Design review of the part shown in the three views and the two pictorial views. Dimensions are in mm from the part's minimum x, y and z. A direction names the side the tool comes from. Coordinates: 2 decimals unless noted, no trailing zeros. Order: outer loops, then holes, each group sorted by start corner. A loop starts at its lowest first (then second) coordinate and runs counter-clockwise, first axis right, second up. Notation, with made-up numbers: (-3.75, 59.5) -> (20.25, 59.5) arc R22 cw to (20.25, 67.5) -> close; hole circle Ø6 at (2.25, 22.5). An arc over 180 degrees is marked (long way). Answer as a JSON object with one key per item and string values. Group by question number.
1) Wall thickness on L1, parallel to X at y = 3.05, z = 22.5; L2, parallel to Z at x = 33, y = 3; L3, parallel to X at y = 4.75, z = 12.75: over which ranges is each line inside the solid? List them lowest first.
2) For pin 1 (1.9 mm diameter, centred on y = 1, z = 12, fed in from +X); pin 2 (0.7 mm diameter, centred on x = 27, y = 1, fed in from -Z); pin 3 (5 mm diameter, centred on x = 33.5, z = 22.5, fed in from -Y), all flat-tipped, find the tip position at first contact; note any pin that passes through.
3) Add section B-B, the plane z = 22.5. Write out the cut boundary in (x, y), then the cut area to 3 significant figures.
4) Add section D-D, the plane z = 1.5. Write out the cut boundary in (x, y), then the cut area to 3 significant figures.
5) Add section A-A, the plane x = 33.5. Write out the cut boundary in (y, z), then the cut area to 3 significant figures.
6) Machinability: for the marked faces 1, 2, 3, 4 and 5, which of the approach directions +Z, -Z, +X, -X, +Y, -Y give a long, thin tool a straight path to every point of the face, cutting with its end or side? Answer none if there is none.
7) Add section C-C, the plane x = 22.5. Write out the cut boundary in (y, z), then the cut area to 3 significant figures.
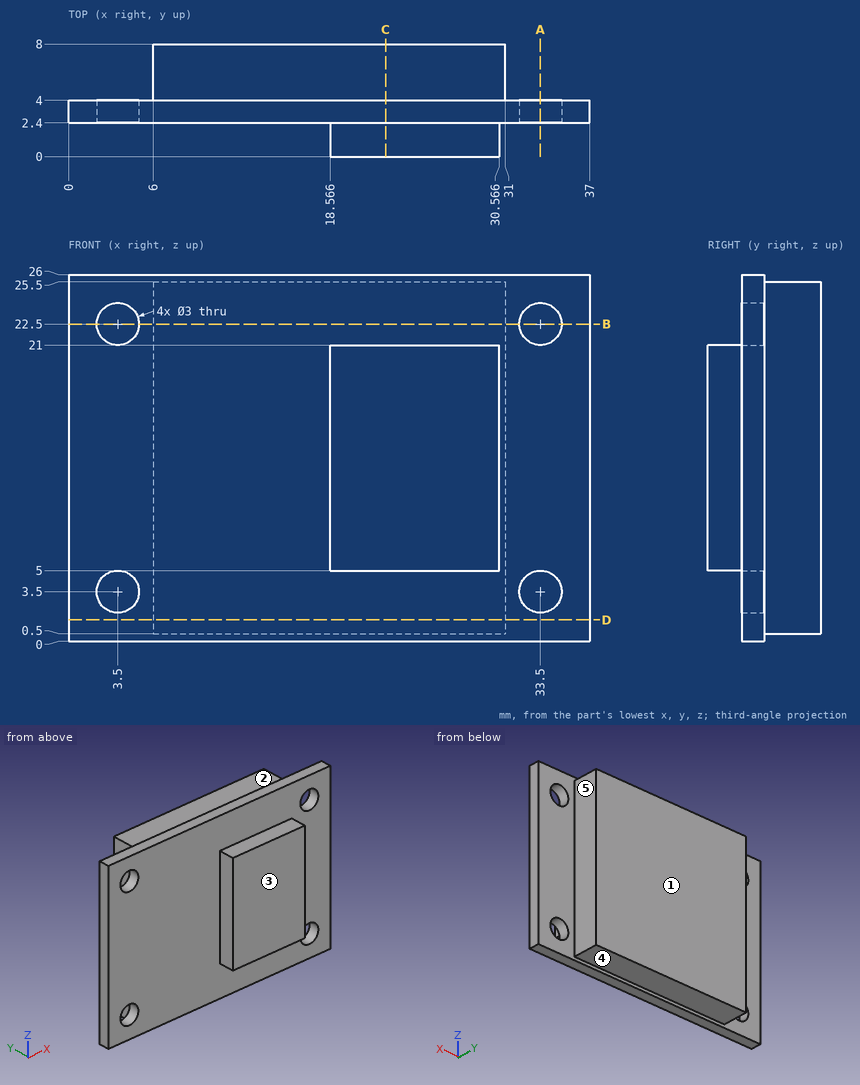
Output values:
{
 "1": {"L1": "x = 0 to 2, 5 to 32, 35 to 37", "L2": "z = 0 to 2.09, 4.91 to 21.09, 23.91 to 26", "L3": "x = 6 to 31"},
 "2": {"pin 1": "stops at x = 30.57", "pin 2": "stops at z = 5", "pin 3": "stops at y = 2.4"},
 "3": {"outline": "(0, 2.4) -> (2, 2.4) -> (2, 4) -> (0, 4) -> close; (5, 2.4) -> (32, 2.4) -> (32, 4) -> (31, 4) -> (31, 8) -> (6, 8) -> (6, 4) -> (5, 4) -> close; (35, 2.4) -> (37, 2.4) -> (37, 4) -> (35, 4) -> close", "area": "150 mm²"},
 "4": {"outline": "(0, 2.4) -> (37, 2.4) -> (37, 4) -> (31, 4) -> (31, 8) -> (6, 8) -> (6, 4) -> (0, 4) -> close", "area": "159 mm²"},
 "5": {"outline": "(2.4, 0) -> (4, 0) -> (4, 2) -> (2.4, 2) -> close; (2.4, 5) -> (4, 5) -> (4, 21) -> (2.4, 21) -> close; (2.4, 24) -> (4, 24) -> (4, 26) -> (2.4, 26) -> close", "area": "32.0 mm²"},
 "6": {"face 1": "+Z, -Z, +X, -X, +Y", "face 2": "+Z, +X, -X, +Y", "face 3": "+Z, -Z, +X, -X, -Y", "face 4": "-Z, +X, -X, +Y", "face 5": "+Z, -Z, +X, +Y"},
 "7": {"outline": "(0, 5) -> (2.4, 5) -> (2.4, 0) -> (4, 0) -> (4, 0.5) -> (8, 0.5) -> (8, 25.5) -> (4, 25.5) -> (4, 26) -> (2.4, 26) -> (2.4, 21) -> (0, 21) -> close", "area": "180 mm²"}
}
